from build123d import *

# Parameters (mm, degrees)
F0_R      = 1.3
F9_DEPTH  = 5.59188
F3_R      = 1.3
F7_R      = 1.3
F8_R      = 1.3
F4_R      = 1.3
F10_DEPTH = 12.5
F11_R     = 5
F12_R     = 7


with BuildPart() as f9:
    # F0 (on Front) → F9 (new body)
    with BuildSketch(Plane.XZ):
        with BuildLine():
            Line((0, 105.927363), (-14.3, 105.927363))
            Line((-14.3, 105.927363), (-14.3, -50.272637))
            Line((-14.3, -50.272637), (17.7, -50.272637))
            Line((17.7, -50.272637), (17.7, -51.772637))
            Line((17.7, -51.772637), (15.2, -51.772637))
            Line((15.2, -51.772637), (15.2, -57.772637))
            Line((15.2, -57.772637), (22.56546, -51.772637))
            Line((22.56546, -51.772637), (22.56546, -41.172637))
            Line((22.56546, -41.172637), (0, -41.172637))
            ThreePointArc((0, -41.172637), (-3.317792, -33.70843), (0, -26.244223))
            ThreePointArc((0, -26.244223), (5.555396, -15.397738), (0, -4.551252))
            ThreePointArc((0, -4.551252), (-5.254266, 2.605622), (-0.450577, 10.072397))
            ThreePointArc((-0.450577, 10.072397), (5.010963, 18.897612), (0, 27.986236))
            ThreePointArc((0, 27.986236), (-3.804451, 34.821723), (0, 41.657209))
            ThreePointArc((0, 41.657209), (4.388049, 49.850428), (0, 58.043648))
            ThreePointArc((0, 58.043648), (-4.094802, 65.3005), (0, 72.557352))
            ThreePointArc((0, 72.557352), (5.764102, 80.860864), (0, 89.164376))
            Line((0, 89.164376), (0, 105.927363))
        make_face()
        with Locations((0, -45.272637)):
            Circle(F0_R, mode=Mode.SUBTRACT)
    extrude(amount=F9_DEPTH)

    # F3 (on face) + F7 (on face) + F8 (on face) + F4 (on face) → F10 (cut, symmetric)
    with BuildSketch(Plane(origin=(0, -3.143985, -0.741469), x_dir=(-1, 0, 0), z_dir=(0, 0.973299, 0.22954))):
        with Locations((0, -13.714992)):
            Circle(F3_R)
    with BuildSketch(Plane(origin=(0, 10.796876, 2.546305), x_dir=(-1, 0, 0), z_dir=(0, 0.973299, 0.22954))):
        with Locations((0, 47.036983)):
            Circle(F7_R)
    with BuildSketch(Plane(origin=(0, 17.767307, 4.190192), x_dir=(-1, 0, 0), z_dir=(0, 0.973299, 0.22954))):
        with Locations((0, 77.403918)):
            Circle(F8_R)
    with BuildSketch(Plane(origin=(0, 3.826445, 0.902418), x_dir=(-1, 0, 0), z_dir=(0, 0.973299, 0.22954))):
        with Locations((0, 16.608408)):
            Circle(F4_R)
    extrude(amount=F10_DEPTH, both=True, mode=Mode.SUBTRACT)

    # F11
    f11_edges = [f9.edges().sort_by_distance(p)[0] for p in [
        (22.56546, -2.79594, -41.172637),
    ]]
    fillet(f11_edges, radius=F11_R)

    # F12
    f12_edges = [f9.edges().sort_by_distance(p)[0] for p in [
        (22.56546, -2.79594, -51.772637),
    ]]
    fillet(f12_edges, radius=F12_R)


solid = f9.part
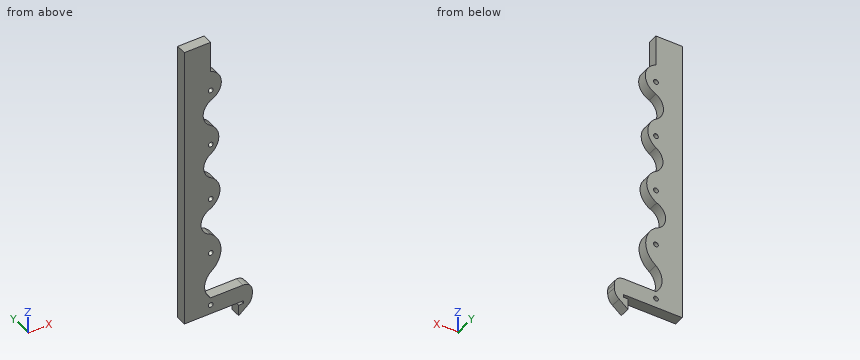
Read the model definition and answer for the solid it produces. Units are mm, in the model's axes. Round coordinates to 2 decimals unless told otherwise and drop trailing zeros. Loops run counter-clockwise (first coordinate to the right, second up) from the corner with the lowest first, then second, coordinate; pieces in that order, holes last.
Q1. Each of these flat-tipped pins is pushed along its axis until it touches: pin 1 (1.7 mm diameter, centred on x = -4, y = -2.5, fed in from -Z); pin 2 (1 mm diameter, centred on y = -4, z = 34, fed in from +X); pin 3 (3 mm diameter, centred on x = 16.5, y = -4, fed in from +Z). Where does it stop, or does it pass through?
Q2. Section A-A on x = -8 is taken. Write down the section's boundary in (y, z).
Q3. Section C-C on z = -23 is taken. Write down the section's boundary in (x, y), and give its area (3 significant figures).
Q4. Section B-B on y = -4.3 is taken. Give the number of separate pieces and of enclosed holes in the cut face, and give its area (3 significant figures).
Q5. Consider probe 1 along Z at (x, y) = (3, -0.95); probe 2 along Z at (x, y) = (13.5, -3.25); probe 3 along Z at (x, y) = (-7, -1.35). Determine where each line is inside the solid, lowest interval first.
Output:
1. pin 1: stops at z = -50.27
1. pin 2: stops at x = -3.7
1. pin 3: stops at z = -41.17
2. outline: (-5.59, -50.27) - (0, -50.27) - (0, 105.93) - (-5.59, 105.93) - close
3. outline: (-14.3, -5.59) - (3.18, -5.59) - (3.18, 0) - (-14.3, 0) - close
3. area: 97.8 mm2
4. separate pieces: 1
4. enclosed holes: 5
4. area: 2,530 mm2
5. probe 1: z = -50.27 to -41.17, -23.26 to -7.54, 13.04 to 25.27, 44.81 to 54.89, 74.43 to 87.29
5. probe 2: z = -50.27 to -41.17
5. probe 3: z = -50.27 to 105.93
